For this review, take the finished solid that the model builds, in its own axes (mm). Face numbers are marked on the shaded views. A direction names the side the tool comes from. Coordinates: 2 decimals unless noted, no trailing zeros. Loops run counter-clockwise (first coordinate to the right, second up) from the corner with the lowest first, then second, coordinate; pieces in that order, holes last.
1. Take a section at A-A, the plane z = -19.5. State the section outline as (x, y) points.
2. Take a section at B-B, the plane y = 6.5. State the section outline as (x, z) points, then the cut area to 3 significant figures.
3. Take a section at C-C, the plane x = 12.5. State the section outline as (y, z) points, then the cut area to 3 significant figures.
4. Mouldability with a two-part tool opening along X and no side actions: class the marked faces 1, 2 and 3 as pulls with the +X half, pulls with the -X half, needs draft (parallel to the pull), parting line crosses it, or undercut.
5. Clearance check with flat-ended pins moving along their axes: P1, Ø2, axis at x = 0, z = -30, coming from the +Y side; P2, Ø1, axis at y = 0.5, z = -29.5, coming from the +X side; P3, Ø2, axis at x = -17, y = 6.5, coming from the -Z side; P4, Ø2, axis at y = 1, z = -29.5, coming from the -X side. State where each tip first meets the part, or that it passes through.
6. Machinability: for the marked faces 4, 5 and 6, which of the approach directions +Z, -Z, +X, -X, +Y, -Y give a long, thin tool a straight path to every point of the face, cutting with its end or side? Answer none if there is none.
7. Take a section at D-D, the plane x = 0. State the section outline as (y, z) points, then the cut area to 3 significant figures.
8. To check wall thickness, follow probe 1 along X at (y, z) = (0.75, -30); probe 2 along X at (y, z) = (0.5, 17); probe 3 along Y at (x, z) = (2.5, -27). State the ranges of each line that lie inside material, in increasing order.
```python
from build123d import *

# Parameters (mm, degrees)
BOSS_EXTRUDE3_DEPTH        = 2
BOSS_EXTRUDE4_START        = 7
BOSS_EXTRUDE4_DEPTH        = 7
F_2_5_2_5_DIAMETER_HOLE2_D = 2.5
M25_CLEARANCE_HOLE2_D      = 28.4
SKETCH27_R                 = 2.8
SKETCH27_R_2               = 2.85
CUT_EXTRUDE7_DEPTH         = 5.5


with BuildPart() as part:
    # Sketch14 → Boss-Extrude3 (new body)
    with BuildSketch(Plane(origin=(0, 2, 0), x_dir=(1, 0, 0), z_dir=(0, 1, 0))):
        with BuildLine():
            Line((-25.401863282, -11.779021258), (-27.230762114, -12.834936491))
            ThreePointArc((-27.230762114, -12.834936491), (-28.145825623, -16.25), (-24.730762114, -17.165063509))
            Line((-24.730762114, -17.165063509), (-22.901863282, -16.109148277))
            ThreePointArc((-22.901863282, -16.109148277), (0, -28), (22.901863282, -16.109148277))
            Line((22.901863282, -16.109148277), (24.730762114, -17.165063509))
            ThreePointArc((24.730762114, -17.165063509), (28.145825623, -16.25), (27.230762114, -12.834936491))
            Line((27.230762114, -12.834936491), (25.401863282, -11.779021258))
            ThreePointArc((25.401863282, -11.779021258), (24.248711306, 14), (2.5, 27.888169535))
            Line((2.5, 27.888169535), (2.5, 30))
            ThreePointArc((2.5, 30), (0, 32.5), (-2.5, 30))
            Line((-2.5, 30), (-2.5, 27.888169535))
            ThreePointArc((-2.5, 27.888169535), (-24.248711306, 14), (-25.401863282, -11.779021258))
        make_face()
    extrude(amount=-BOSS_EXTRUDE3_DEPTH)

    # Sketch15 → Boss-Extrude4 (add)
    with BuildSketch(Plane(origin=(0, 2, 0), x_dir=(-1, 0, 0), z_dir=(0, 1, 0)).offset(BOSS_EXTRUDE4_START)):
        with BuildLine():
            Line((-20.2, -6.36507512), (18.8, -6.36507512))
            ThreePointArc((18.8, -6.36507512), (23.327173423, -8.462287904), (24.654830029, -13.271750307))
            ThreePointArc((24.654830029, -13.271750307), (23.430757061, -15.329697439), (22.035331707, -17.275536361))
            ThreePointArc((22.035331707, -17.275536361), (21.029921495, -17.800071223), (19.943097949, -18.123801199))
            Line((19.943097949, -18.123801199), (-21.343097949, -18.123801199))
            ThreePointArc((-21.343097949, -18.123801199), (-23.915273063, -14.562270232), (-25.898699677, -10.64224389))
            ThreePointArc((-25.898699677, -10.64224389), (-23.762630724, -7.553317405), (-20.2, -6.36507512))
        make_face()
    extrude(amount=-BOSS_EXTRUDE4_DEPTH)

    # Ø2.5 (2.5) Diameter Hole2 (through all)
    with Locations(Plane(origin=(0, 2, 0), x_dir=(1, 0, 0), z_dir=(0, 1, 0))):
        with Locations((-25.980762114, -15), (25.980762114, -15), (0, 30)):
            Hole(F_2_5_2_5_DIAMETER_HOLE2_D / 2)

    # M25 Clearance Hole2 (through all)
    with Locations(Plane(origin=(0, 0, 0), x_dir=(-1, 0, 0), z_dir=(0, -1, 0))):
        with Locations((-0.7, 12.3)):
            Hole(M25_CLEARANCE_HOLE2_D / 2)

    # Sketch27 → Cut-Extrude7 (cut)
    with BuildSketch(Plane(origin=(0, 9, 0), x_dir=(1, 0, 0), z_dir=(0, 1, 0))):
        with Locations(Location((-18.398233243, 12.782862889, 0), (0, 0, 270))):
            Circle(SKETCH27_R)
        with Locations(Location((20.562204281, 12.782862889, 0), (0, 0, 270))):
            Circle(SKETCH27_R_2)
    extrude(amount=-CUT_EXTRUDE7_DEPTH, mode=Mode.SUBTRACT)


solid = part.part
```
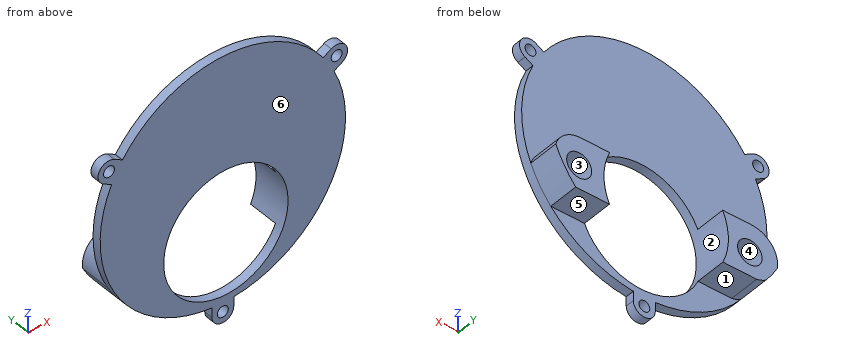
Results list:
1. outline: (-20.09, 0) - (-11.54, 0) - (-11.54, 2) - (-20.09, 2) - close; (12.94, 0) - (20.09, 0) - (20.09, 2) - (12.94, 2) - close
2. outline: (-24.65, -13.27) arc R28 ccw to (-22.04, -17.28) arc R5.93 ccw to (-19.94, -18.12) - (-12.25, -18.12) arc R14.2 cw to (-12.2, -6.37) - (-18.8, -6.37) arc R5.93 ccw to start; (13.6, -6.37) arc R14.2 cw to (13.65, -18.12) - (21.34, -18.12) arc R28 ccw to (25.9, -10.64) arc R5.93 ccw to (20.2, -6.37) - close; hole circle Ø5.6 at (-18.4, -12.78); hole circle Ø5.7 at (20.56, -12.78)
2. area: 184 mm2
3. outline: (0, -25.05) - (2, -25.05) - (2, -20.2) - (0, -20.2) - close; (0, -4.4) - (2, -4.4) - (2, 25.05) - (0, 25.05) - close
3. area: 68.6 mm2
4. face 1: needs draft
4. face 2: undercut
4. face 3: undercut
5. P1: passes through
5. P2: stops at x = 2.5
5. P3: stops at z = -18.12
5. P4: stops at x = -2.5
6. face 4: +Y
6. face 5: -Z, +X, -X, +Y
6. face 6: +Z, -Z, +X, -X, -Y
7. outline: (0, -32.5) - (2, -32.5) - (2, -31.25) - (0, -31.25) - close; (0, -28.75) - (2, -28.75) - (2, -26.48) - (0, -26.48) - close; (0, 1.88) - (2, 1.88) - (2, 28) - (0, 28) - close
7. area: 59.3 mm2
8. probe 1: x = -2.5 to -1.25, 1.25 to 2.5
8. probe 2: x = -27.48 to -24.44, -22.25 to 22.25, 24.44 to 27.48
8. probe 3: y = 0 to 2
